Check sheet for the modelled part. Datum: model origin and axes. Units: mm. A direction names the side the tool comes from. Round coordinates to 2 decimals unless told otherwise and drop trailing zeros. Order: outer loops, then holes, each group sorted by start corner. A loop starts at its lowest first (then second) coordinate and runs counter-clockwise, first axis right, second up.
from build123d import *

# Parameters (mm, degrees)
BOSS_EXTRUDE1_DEPTH          = 7
CUT_EXTRUDE1_DEPTH           = 4
CUT_EXTRUDE4_DEPTH           = 30.03484975
SKETCH8_R                    = 2
CUT_EXTRUDE5_DEPTH           = 18
SKETCH9_R                    = 3
CUT_EXTRUDE6_DEPTH           = 8.1
SKETCH10_W                   = 40
SKETCH10_H                   = 6.5
CUT_EXTRUDE7_DEPTH           = 30.034849842
FILLET1_R                    = 2
SKETCH11_R                   = 1.5
CUT_EXTRUDE8_DEPTH           = 3
CUT_EXTRUDE8_DRAFT           = -20
CUT_EXTRUDE8_PROFILE_2_DEPTH = 3
CUT_EXTRUDE8_PROFILE_2_DRAFT = -20
CUT_EXTRUDE8_PROFILE_3_DEPTH = 3
CUT_EXTRUDE8_PROFILE_3_DRAFT = -20


with BuildPart() as part:
    # Sketch1 → Boss-Extrude1 (new body)
    with BuildSketch(Plane.XY):
        with BuildLine():
            Line((0, 0), (18, 0))
            ThreePointArc((18, 0), (19.414213562, 0.585786438), (20, 2))
            Line((20, 2), (20, 11.945768163))
            ThreePointArc((20, 11.945768163), (19.769252649, 12.878369398), (19.130254936, 13.595775369))
            Line((19.130254936, 13.595775369), (10.510938386, 19.500007206))
            ThreePointArc((10.510938386, 19.500007206), (9.972285338, 19.760499203), (9.380683449, 19.85))
            Line((9.380683449, 19.85), (-9.380683449, 19.85))
            ThreePointArc((-9.380683449, 19.85), (-9.972285338, 19.760499203), (-10.510938386, 19.500007206))
            Line((-10.510938386, 19.500007206), (-19.130254936, 13.595775369))
            ThreePointArc((-19.130254936, 13.595775369), (-19.769252649, 12.878369398), (-20, 11.945768163))
            Line((-20, 11.945768163), (-20, 2))
            ThreePointArc((-20, 2), (-19.414213562, 0.585786438), (-18, 0))
            Line((-18, 0), (0, 0))
        make_face()
        with BuildLine():
            Line((-13.75, 9.075), (-13.75, 4.625))
            ThreePointArc((-13.75, 4.625), (-15.375, 3), (-17, 4.625))
            Line((-17, 4.625), (-17, 9.075))
            ThreePointArc((-17, 9.075), (-15.375, 10.7), (-13.75, 9.075))
        make_face(mode=Mode.SUBTRACT)
        with BuildLine():
            Line((17, 9.075), (17, 4.625))
            ThreePointArc((17, 4.625), (15.375, 3), (13.75, 4.625))
            Line((13.75, 4.625), (13.75, 9.075))
            ThreePointArc((13.75, 9.075), (15.375, 10.7), (17, 9.075))
        make_face(mode=Mode.SUBTRACT)
    extrude(amount=BOSS_EXTRUDE1_DEPTH)

    # Sketch2 → Cut-Extrude1 (cut)
    with BuildSketch(Plane.XY.offset(7)):
        with BuildLine():
            Line((-18.375, 4.625), (-18.375, 9.075))
            ThreePointArc((-18.375, 9.075), (-15.375, 12.075), (-12.375, 9.075))
            Line((-12.375, 9.075), (-12.375, 4.625))
            ThreePointArc((-12.375, 4.625), (-15.375, 1.625), (-18.375, 4.625))
        make_face()
        with BuildLine():
            Line((12.375, 4.625), (12.375, 9.075))
            ThreePointArc((12.375, 9.075), (15.375, 12.075), (18.375, 9.075))
            Line((18.375, 9.075), (18.375, 4.625))
            ThreePointArc((18.375, 4.625), (15.375, 1.625), (12.375, 4.625))
        make_face()
    extrude(amount=-CUT_EXTRUDE1_DEPTH, mode=Mode.SUBTRACT)

    # Sketch6 → Cut-Extrude4 (cut, through all)
    with BuildSketch(Plane.XY.offset(7)):
        Polygon((-13.5, 13.35), (-6.5, 13.35), (-6.5, 19.85), (6.5, 19.85), (6.5, 13.35), (13.5, 13.35), (13.5, 11.75), (-13.5, 11.75), align=None)
    extrude(amount=-CUT_EXTRUDE4_DEPTH, mode=Mode.SUBTRACT)

    # Sketch8 → Cut-Extrude5 (cut)
    with BuildSketch(Plane(origin=(0, 19.85, 0), x_dir=(1, 0, 0), z_dir=(0, 1, 0))):
        with Locations(Location((-10, -3.5, 0), (0, 0, 180))):
            Circle(SKETCH8_R)
        with Locations(Location((10, -3.5, 0), (0, 0, 180))):
            Circle(SKETCH8_R)
    extrude(amount=-CUT_EXTRUDE5_DEPTH, mode=Mode.SUBTRACT)

    # Sketch9 → Cut-Extrude6 (cut)
    with BuildSketch(Plane(origin=(0, 19.85, 0), x_dir=(1, 0, 0), z_dir=(0, 1, 0))):
        with Locations(Location((10, -3.5, 0), (0, 0, 101.913740948))):
            Circle(SKETCH9_R)
        with Locations(Location((-10, -3.5, 0), (0, 0, 99.806006121))):
            Circle(SKETCH9_R)
    extrude(amount=-CUT_EXTRUDE6_DEPTH, mode=Mode.SUBTRACT)

    # Sketch10 → Cut-Extrude7 (cut, through all)
    with BuildSketch(Plane.XY.offset(7)):
        with Locations((0, 16.6)):
            Rectangle(SKETCH10_W, SKETCH10_H)
    extrude(amount=-CUT_EXTRUDE7_DEPTH, mode=Mode.SUBTRACT)

    # Fillet1
    # the kernel refuses this fillet: 2 mm, written as the material it takes off along each edge
    with BuildSketch(Plane(origin=(-19.424125327, 13.35, 12.203143064), x_dir=(-0.27669557885699486, -0.9609576247894558, 0), z_dir=(0, 0, -1))) as fillet1_piece_1:
        with BuildLine():
            CenterArc((1.527866068, -1.92191525), FILLET1_R, 73.936914891, 90)
            Line((-0.394049182, -1.368524092), (-0.586240707, -1.313184976))
            Line((-0.586240707, -1.313184976), (-0.192191525, 0.055339116))
            Line((-0.192191525, 0.055339116), (-0.095535811, 0.175706883))
            ThreePointArc((-0.095535811, 0.175706883), (1.564088383, 0.357037942), (2.136596341, 0.192191525))
            Line((2.136596341, 0.192191525), (2.081257226, 0))
        make_face()
    extrude(amount=17.406286128, mode=Mode.SUBTRACT)
    with BuildSketch(Plane(origin=(19.424125327, 13.35, 12.203143064), x_dir=(-1, 0, 0), z_dir=(0, 0, -1))) as fillet1_piece_2:
        with BuildLine():
            CenterArc((1.424125327, -2), FILLET1_R, 90, 90)
            Line((-0.575874673, -2), (-0.775874673, -2))
            ThreePointArc((-0.775874673, -2), (-0.775874673, -1.404231837), (-0.142412533, 0.140423184))
            Line((-0.142412533, 0.140423184), (0, 0.2))
            Line((0, 0.2), (1.424125327, 0.2))
            Line((1.424125327, 0.2), (1.424125327, 0))
        make_face()
    extrude(amount=17.406286128, mode=Mode.SUBTRACT)


with BuildPart() as cut_extrude8_tool:
    # Sketch11 → Cut-Extrude8 (with draft: the straight prism first)
    with BuildSketch(Plane(origin=(0, 11.75, 0), x_dir=(1, 0, 0), z_dir=(0, 1, 0))):
        with Locations((0, -3.5)):
            Circle(SKETCH11_R)
    extrude(amount=-CUT_EXTRUDE8_DEPTH)
    # Cut-Extrude8: the draft: its side faces are tilted about the plane it starts from
    cut_extrude8_sides = [cut_extrude8_tool.faces().sort_by_distance(p)[0] for p in [
        (-1.5, 10.25, 3.5),
    ]]
    draft(cut_extrude8_sides, Plane(origin=(0, 11.75, 0), x_dir=(1, 0, 0), z_dir=(0, 1, 0)), CUT_EXTRUDE8_DRAFT)


with BuildPart() as part_1:
    add(part.part)

    # Cut-Extrude8: cut by cut_extrude8_tool
    add(cut_extrude8_tool.part, mode=Mode.SUBTRACT)


with BuildPart() as cut_extrude8_profile_2_tool:
    # Sketch11 → Cut-Extrude8 profile 2 (with draft: the straight prism first)
    with BuildSketch(Plane(origin=(0, 11.75, 0), x_dir=(1, 0, 0), z_dir=(0, 1, 0))):
        with Locations((5, -3.5)):
            Circle(SKETCH11_R)
    extrude(amount=-CUT_EXTRUDE8_PROFILE_2_DEPTH)
    # Cut-Extrude8 profile 2: the draft: its side faces are tilted about the plane it starts from
    cut_extrude8_profile_2_sides = [cut_extrude8_profile_2_tool.faces().sort_by_distance(p)[0] for p in [
        (3.5, 10.25, 3.5),
    ]]
    draft(cut_extrude8_profile_2_sides, Plane(origin=(0, 11.75, 0), x_dir=(1, 0, 0), z_dir=(0, 1, 0)), CUT_EXTRUDE8_PROFILE_2_DRAFT)


with BuildPart() as part_2:
    add(part_1.part)

    # Cut-Extrude8 profile 2: cut by cut_extrude8_profile_2_tool
    add(cut_extrude8_profile_2_tool.part, mode=Mode.SUBTRACT)


with BuildPart() as cut_extrude8_profile_3_tool:
    # Sketch11 → Cut-Extrude8 profile 3 (with draft: the straight prism first)
    with BuildSketch(Plane(origin=(0, 11.75, 0), x_dir=(1, 0, 0), z_dir=(0, 1, 0))):
        with Locations((-5, -3.5)):
            Circle(SKETCH11_R)
    extrude(amount=-CUT_EXTRUDE8_PROFILE_3_DEPTH)
    # Cut-Extrude8 profile 3: the draft: its side faces are tilted about the plane it starts from
    cut_extrude8_profile_3_sides = [cut_extrude8_profile_3_tool.faces().sort_by_distance(p)[0] for p in [
        (-6.5, 10.25, 3.5),
    ]]
    draft(cut_extrude8_profile_3_sides, Plane(origin=(0, 11.75, 0), x_dir=(1, 0, 0), z_dir=(0, 1, 0)), CUT_EXTRUDE8_PROFILE_3_DRAFT)


with BuildPart() as part_3:
    add(part_2.part)

    # Cut-Extrude8 profile 3: cut by cut_extrude8_profile_3_tool
    add(cut_extrude8_profile_3_tool.part, mode=Mode.SUBTRACT)


solid = part_3.part
1) Gauge pin test, flat ends, axial feed: pin 1 (3.5 mm diameter, centred on x = -10, z = 3.5, fed in from +Y); pin 2 (1.8 mm diameter, centred on y = 12.5, z = 3.5, fed in from +X); pin 3 (1.8 mm diameter, centred on x = 17, y = 5.5, fed in from +Z). Record the tip position at first contact, or that the pin passes through.
2) Scan lines: line 1 (Z direction, x = 10, y = 9.5); line 2 (X direction, y = 2, z = 2.5); line 3 (X direction, y = 9, z = 4.75) (3 decimals). Record each from-to range of solid material in increasing order.
3) Sectioned sample at B-B on z = 1. Record the cut outline in (x, y) (3 decimals).
4) Sectioned sample at D-D on x = 10. Record the cut outline in (y, z), and give its area (4 significant figures).
5) Sectioned sample at A-A on y = 5.25. Record the cut outline in (x, z) (3 decimals), and give its area (3 significant figures).
6) Sectioned sample at C-C on x = 0. Record the cut outline in (y, z), and give its area (3 significant figures).
7) Set-up check for faces 1 (the face through (-18.375, 7, 5)), 2 (the face through (3, 11.75, 4)), 3 (the face through (-17, 7, 1)), 4 (the face through (-10, 1.85, 4)): record each of +Z, -Z, +X, -X, +Y, -Y from which the full face is reachable in a straight line by a thin tool's end or side.
8) Draft check along X on faces 5 (the face through (0, 7, 0)), 6 (the face through (18.375, 7, 5)), 7 (the face through (-20, 7, 3)). Enter one of: pulls with the +X half, pulls with the -X half, needs draft (parallel to the pull), parting line crosses it, or undercut.
Values found:
1. pin 1: stops at y = 1.85
1. pin 2: stops at x = 19.98
1. pin 3: stops at z = 3
2. line 1: z = 0 to 1.5, 5.5 to 7
2. line 2: x = -20 to -11.73, -8.27 to 8.27, 11.73 to 20
2. line 3: x = -20 to -18.375, -12.375 to -11.561, -8.439 to 8.439, 11.561 to 12.375, 18.375 to 20
3. outline: (-20, 2) arc R2 ccw to (-18, 0) - (18, 0) arc R2 ccw to (20, 2) - (20, 11.35) arc R2 ccw to (18, 13.35) - (13.5, 13.35) - (13.5, 11.75) - (-13.5, 11.75) - (-13.5, 13.35) - (-18, 13.35) arc R2 ccw to (-20, 11.35) - close; hole (-17, 4.625) arc R1.625 ccw to (-13.75, 4.625) - (-13.75, 9.075) arc R1.625 ccw to (-17, 9.075) - close; hole (13.75, 4.625) arc R1.625 ccw to (17, 4.625) - (17, 9.075) arc R1.625 ccw to (13.75, 9.075) - close
4. outline: (0, 0) - (11.75, 0) - (11.75, 1.5) - (1.85, 1.5) - (1.85, 5.5) - (11.75, 5.5) - (11.75, 7) - (0, 7) - close
4. area: 42.65 mm2
5. outline: (-20, 0) - (-17, 0) - (-17, 3) - (-18.375, 3) - (-18.375, 7) - (-20, 7) - close; (-13.75, 0) - (13.75, 0) - (13.75, 3) - (12.375, 3) - (12.375, 7) - (-12.375, 7) - (-12.375, 3) - (-13.75, 3) - close; (17, 0) - (20, 0) - (20, 7) - (18.375, 7) - (18.375, 3) - (17, 3) - close; hole circle Ø4 at (-10, 3.5); hole circle Ø4 at (10, 3.5)
5. area: 187 mm2
6. outline: (0, 0) - (11.75, 0) - (11.75, 2) - (8.75, 3.09) - (8.75, 3.91) - (11.75, 5) - (11.75, 7) - (0, 7) - close
6. area: 76.5 mm2
7. face 1: +Z
7. face 2: +Z, -Z, +Y
7. face 3: +Z, -Z
7. face 4: +Y
8. face 5: needs draft
8. face 6: undercut
8. face 7: pulls with the -X half
